Autodesk Inventor part; units mm, degrees
ref_plane "YZ Plane" through (0, 0, 0) normal (1, 0, 0) x (0, 1, 0)
ref_plane "XZ Plane" through (0, 0, 0) normal (0, 1, 0) x (-1, 0, 0)
ref_plane "XY Plane" through (0, 0, 0) normal (0, 0, 1) x (1, 0, 0)
sketch "Sketch1" plane through (0, 0, 0) normal (0, 1, 0) x (-1, 0, 0)
  line L0 (0, 4) -> (0, 8)
  line L1 (0, 8) -> (4.8, 8)
  line L2 (4.8, 8) -> (4.8, 6)
  line L3 (4.8, 6) -> (9.4, 6)
  line L4 (9.4, 6) -> (9.4, 8)
  line L5 (9.4, 8) -> (38.2679, 8)
  line L6 (0, 4) -> (7.5, 4)
  line L7 (7.5, 4) -> (7.5, 3.25)
  line L8 (40, 4) -> (36.8, 4)
  line L9 (36.8, 4) -> (36.8, 3.25)
  line L10 (40, 4) -> (40, 5)
  line L11 (38.2679, 8) -> (40, 5)
  line L12 (36.8, 3.25) -> (7.5, 3.25)
  line L13 (0, 0) -> (40, 0) construction
  dimension "d0" = 8
  dimension "d1" = 4.8
  dimension "d3" = 4.6
  dimension "d10" = 2
  dimension "d11" = 2
  dimension "d12" = 7.5
  dimension "d13" = 4
  dimension "d14" = 3.25
  dimension "d15" = 3.2
  dimension "d16" = 4
  dimension "d19" = 3.25
  dimension "d20" = 120
  dimension "d21" = 40
  dimension "d22" = 5
  dimension "d23" = 40
revolve "Revolution1" add sketch "Sketch1" angle 360 about axis through (0, 0, 0) along (-1, 0, 0)
properties part number "NozzleHolder" material "Polyethylene, High Density"
For this review, take the finished solid that the model builds, in its own axes (mm). A direction names the side the tool comes from. Coordinates: 2 decimals unless noted, no trailing zeros. Order: outer loops, then holes, each group sorted by start corner. A loop starts at its lowest first (then second) coordinate and runs counter-clockwise, first axis right, second up. Notation, with made-up numbers: (70, 72.5) -> (100, 72.5) arc R20 ccw to (100, 93.5) -> close; hole circle Ø8 at (43, 15). An arc over 180 degrees is marked (long way). Return JSON: item names as keys, results as strings.
1. For pin 1 Ø7 at (y, z) = (0, 0) entering from -X; pin 2 Ø1 at (x, z) = (-18.5, -1) entering from +Y; pin 3 Ø7 at (y, z) = (0, 0) entering from +X, all flat-tipped, find the tip position at first contact; note any pin that passes through.
Answer block:
{"pin 1": "x = -36.8", "pin 2": "y = 7.98", "pin 3": "x = -7.5"}
2. We need section C-C on x = -11. Write out the cut boundary in (y, z), and give its area (3 significant figures).
Answer block:
{"outline": "circle Ø16 at (0, 0); hole circle Ø6.5 at (0, 0)", "area": "168 mm²"}
3. Machinability: for faces 1 (the flat face through (-4.8, 6, -2)), 2 (the flat face through (-7.5, 3, -2)), 3 (the cylindrical face through (-2.43, -7.81, -1.73)), 4 (the flat face through (0, -2, -4)), 5 (the cylindrical face through (-38.378, 3.905, -0.867)), which of the approach directions +Z, -Z, +X, -X, +Y, -Y give a long, thin tool a straight path to every point of the face, cutting with its end or side? Answer none if there is none.
Answer block:
{"face 1": "none", "face 2": "+X", "face 3": "+X, -X", "face 4": "+Z, -Z, +X, +Y, -Y", "face 5": "-X"}
4. We need section A-A on z = 0. Write out the cut boundary in (x, y).
Answer block:
{"outline": "(-40, -5) -> (-38.27, -8) -> (-9.4, -8) -> (-9.4, -6) -> (-4.8, -6) -> (-4.8, -8) -> (0, -8) -> (0, -4) -> (-7.5, -4) -> (-7.5, -3.25) -> (-36.8, -3.25) -> (-36.8, -4) -> (-40, -4) -> close; (-40, 4) -> (-36.8, 4) -> (-36.8, 3.25) -> (-7.5, 3.25) -> (-7.5, 4) -> (0, 4) -> (0, 8) -> (-4.8, 8) -> (-4.8, 6) -> (-9.4, 6) -> (-9.4, 8) -> (-38.27, 8) -> (-40, 5) -> close"}
5. For line 1 (Y direction, x = -24, z = 0); line 2 (Y direction, x = -1.5, z = 0.25); line 3 (Z direction, x = -11, y = -0.25), list the stretches that pass through material, from the lowest coordinate up. Write a range as from..to.
Answer block:
{"line 1": "-8..-3.25, 3.25..8", "line 2": "-8..-3.99, 3.99..8", "line 3": "-8..-3.24, 3.24..8"}
6. The part is to be moulded in two halves that separate along X. For faces 6 (the conical face through (-39.892, 5.064, -1.125)), 7 (the cylindrical face through (-24.04, -7.81, -1.73)), 8 (the flat face through (-9.4, 6, -2)), say which applies: +X half, -X half, draft (parallel to the pull), parting line (faces both ways), or undercut.
Answer block:
{"face 6": "-X half", "face 7": "draft", "face 8": "undercut"}
